Geometry: see drawing. Coordinates: mm, zero at the bounding-box minimum. A direction names the side the tool comes from. Coordinates: 2 decimals unless noted, no trailing zeros. Loops run counter-clockwise (first coordinate to the right, second up) from the corner with the lowest first, then second, coordinate; pieces in that order, holes last.
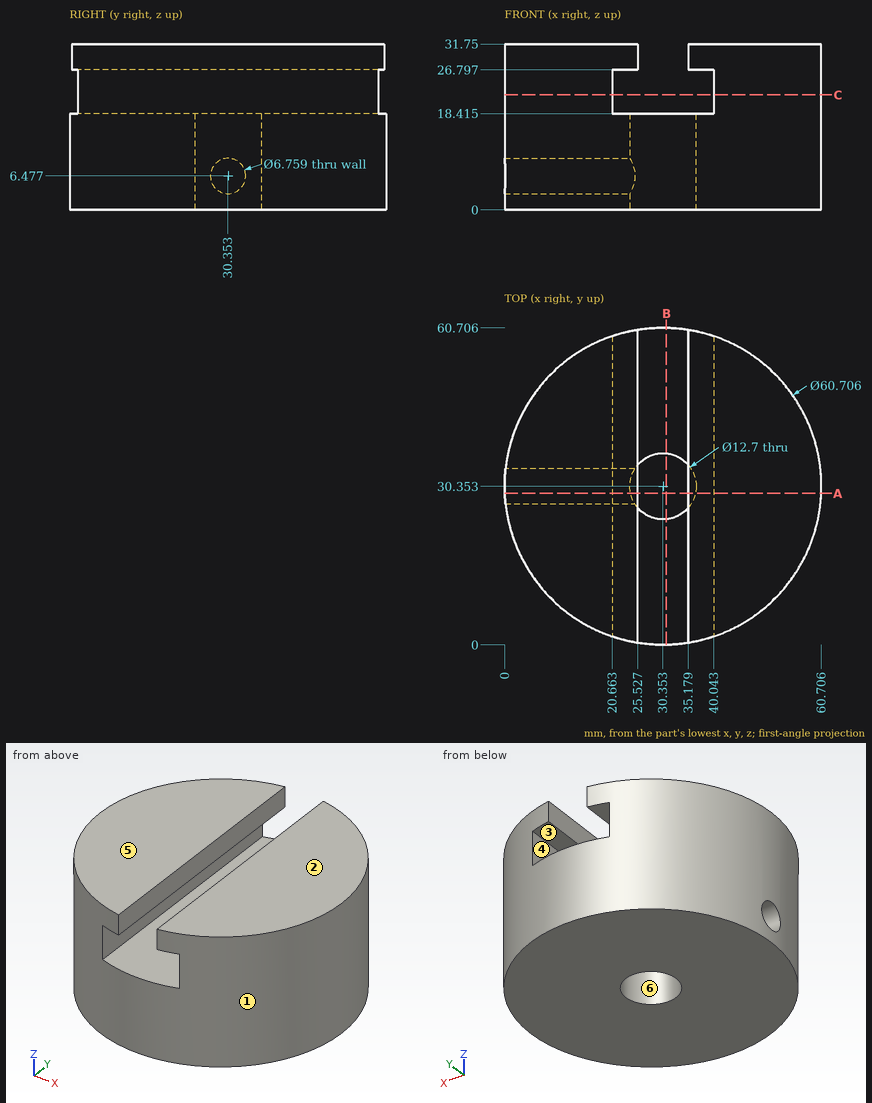
Item 1: Contact query for flat-ended pins moving along their axis: P1, Ø12, axis at x = 6.5, z = 9, coming from the -Y side (1 decimal); P2, Ø10, axis at x = 30.353, y = 30.353, coming from the +Z side; P3, Ø2.5, axis at y = 24, z = 21, coming from the -X side; P4, Ø1.5, axis at y = 40.5, z = 29, coming from the -X side. Output: stop coordinate, or through.
Result:
P1: stops at y = 5.8
P2: stops at z = 31.75
P3: stops at x = 0.43
P4: stops at x = 1.49
Item 2: Section query C-C (z = 22). Output: boundary loops of the cut face in (x, y).
Result:
outline: (20.66, 1.59) - (20.66, 59.12) arc R30.35 ccw to start; (40.04, 1.59) arc R30.35 ccw to (40.04, 59.12) - close
Item 3: Mould query, pull axis X, two halves, no side actions, for the marked faces 1, 2 and 3. Classes: +X half, -X half, draft (parallel to the pull), parting line (faces both ways), or undercut.
Result:
face 1: parting line
face 2: draft
face 3: undercut
Item 4: Section query B-B (x = 31). Output: boundary loops of the cut face in (y, z) (1 decimal).
Result:
outline: (0, 0) - (24, 0) - (24, 18.4) - (0, 18.4) - close; (36.7, 0) - (60.7, 0) - (60.7, 18.4) - (36.7, 18.4) - close
Item 5: Reachability of the marked faces 4, 5 and 6 from +Z, -Z, +X, -X, +Y, -Y: full face, straight path, thin tool, end or side. Return the list, or none.
Result:
face 4: +Y, -Y
face 5: +Z, +X, -X, +Y, -Y
face 6: -Z
Item 6: Line query: L1, parallel to Y at x = 8.5, z = 5 (1 decimal); L2, parallel to X at y = 49.5, z = 30 (1 decimal); L3, parallel to Z at x = 27, y = 38 (1 decimal). Output: solid intervals per line, ascending.
Result:
L1: y = 9.3 to 27.3, 33.4 to 51.4
L2: x = 6.8 to 25.5, 35.2 to 53.9
L3: z = 0 to 18.4
Item 7: Section query A-A (y = 29). Count the separate pieces of the cut face and the enclosed holes in it, then the cut area to 3 significant figures.
Result:
separate pieces: 3
enclosed holes: 0
area: 1,340 mm2
